Read the model definition and answer for the solid it produces. Units are mm, in the model's axes. Face numbers are marked on the shaded views. A direction names the side the tool comes from. Coordinates: 2 decimals unless noted, no trailing zeros. Write each loop counter-clockwise with the first axis right and the second up, starting at its lowest first coordinate (ties: lowest second). Pieces come first, ordered by that corner, then holes.
1) Each of these flat-tipped pins is pushed along its axis until it touches: pin 1 Ø5 at (x, z) = (11.5, 16) entering from +Y; pin 2 Ø10 at (x, y) = (12.5, -15.5) entering from -Z; pin 3 Ø1.5 at (x, z) = (4.5, 10) entering from +Y; pin 4 Ø4 at (x, z) = (0, 18.5) entering from -Y. Where does it stop, or does it pass through?
2) The part is cut by section B-B (z = 25). Give the number of separate pieces and of enclosed holes in the cut face, then the cut area to 3 significant figures.
3) The part is cut by section D-D (x = 0). Determine the outline of the cut face in (y, z).
4) The part is cut by section C-C (y = 6). Determine the outline of the cut face in (x, z), then the cut area to 3 significant figures.
5) Find the intervals of material crossed by line 1 (Y direction, x = 0, z = 23.75); line 2 (Z direction, x = -4.5, y = -4); line 3 (X direction, y = 13, z = 24), in increasing order.
6) The part is cut by section A-A (y = -14.5). Determine the outline of the cut face in (x, z), then the cut area to 3 significant figures.
7) Which of the six approach directions +Z, -Z, +X, -X, +Y, -Y give full straight-line access (tool end or side, diameter ignored) to the marked faces 4 and 5?
8) Determine the mould class of the marked faces 1, 2 and 3 for opening direction Y: +Y half, -Y half, draft (parallel to the pull), parting line (faces both ways), or undercut.
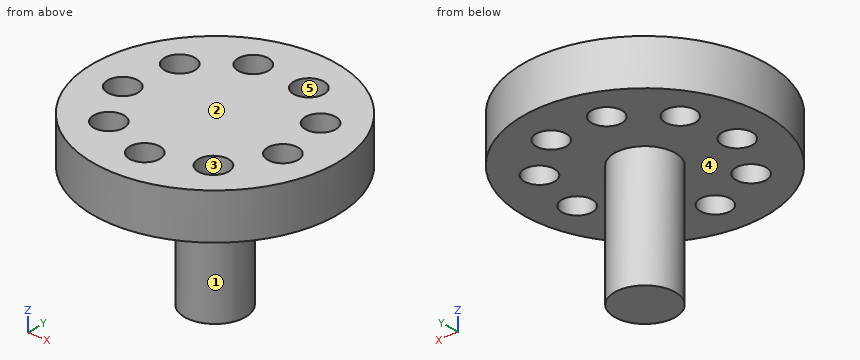
from build123d import *

# Parameters (mm, degrees)
SKETCH001_R        = 2.5
POCKET_DEPTH       = 7.5
POLARPATTERN_COUNT = 9


with BuildPart() as part:
    # Sketch → Revolution (revolve)
    with BuildSketch(Plane.XZ):
        Polygon((0, 0), (5, 0), (5, 20), (20, 20), (20, 27.5), (0, 27.5), align=None)
    revolve(axis=Axis((0, 0, 0), (0, 0, 1)))

    # Sketch001 (on Face5 of Revolution) → Pocket (cut)
    with BuildSketch(Plane(origin=(0, 0, 27.5), x_dir=(-1, 0, 0), z_dir=(0, 0, 1))):
        with Locations((0.017617, 13.499989)):
            Circle(SKETCH001_R)
    pocket = extrude(amount=-POCKET_DEPTH, mode=Mode.SUBTRACT)

    # PolarPattern: Pocket ×9 about axis
    polarpattern_axis = Axis((0, 0, 27.5), (0, 0, 1))
    for i in range(1, POLARPATTERN_COUNT):
        add(pocket.rotate(polarpattern_axis, i * 360 / POLARPATTERN_COUNT), mode=Mode.SUBTRACT)


solid = part.part
Reported:
1. pin 1: passes through
1. pin 2: stops at z = 20
1. pin 3: stops at y = 3.31
1. pin 4: stops at y = -20
2. separate pieces: 1
2. enclosed holes: 9
2. area: 1,080 mm2
3. outline: (-20, 20) - (-16, 20) - (-16, 27.5) - (-20, 27.5) - close; (-11, 20) - (-5, 20) - (-5, 0) - (5, 0) - (5, 20) - (20, 20) - (20, 27.5) - (-11, 27.5) - close
4. outline: (-19.08, 20) - (-14.06, 20) - (-14.06, 27.5) - (-19.08, 27.5) - close; (-9.3, 20) - (9.31, 20) - (9.31, 27.5) - (-9.3, 27.5) - close; (14.09, 20) - (19.08, 20) - (19.08, 27.5) - (14.09, 27.5) - close
4. area: 215 mm2
5. line 1: y = -20 to -16, -11 to 20
5. line 2: z = 20 to 27.5
5. line 3: x = -15.2 to -7.08, -2.12 to 2.15, 7.11 to 15.2
6. outline: (-13.77, 20) - (-2.31, 20) - (-2.31, 27.5) - (-13.77, 27.5) - close; (2.27, 20) - (13.77, 20) - (13.77, 27.5) - (2.27, 27.5) - close
6. area: 172 mm2
7. face 4: -Z
7. face 5: +Z, -Z
8. face 1: parting line
8. face 2: draft
8. face 3: undercut
